Input: part model. Units: mm. Frame: model coordinates. A direction names the side the tool comes from. Give positions to 0.01 mm unless a question says otherwise; leave off trailing zeros. Write each loop counter-clockwise with the first axis right and the second up, starting at its lowest first coordinate (ties: lowest second). Pieces come first, ordered by that corner, then holes.
```python
from build123d import *

# Parameters (mm, degrees)
SALIENTE_EXTRUIR1_START      = 0.1
SALIENTE_EXTRUIR1_DEPTH      = 1.3
SALIENTE_EXTRUIR2_START      = 0.1
SALIENTE_EXTRUIR2_DEPTH      = 1.3
SALIENTE_EXTRUIR2_DEPTH_BACK = 6.6
CROQUIS2_W                   = 45.7
CROQUIS2_H                   = 27.4
CROQUIS2_R                   = 1.65
CROQUIS2_R_2                 = 1.6
SALIENTE_EXTRUIR3_DEPTH      = 5.5
REDONDEO1_R                  = 3


with BuildPart() as part:
    # Croquis1 → Saliente-Extruir1 (new body)
    with BuildSketch(Plane.XY.offset(SALIENTE_EXTRUIR1_START)):
        with BuildLine():
            Line((-105.35, -3.3), (-105.35, -9.05))
            Line((-105.35, -9.05), (-94.282475165, -9.05))
            ThreePointArc((-94.282475165, -9.05), (-93.803420224, -6.334895379), (-91.5, -7.85))
            ThreePointArc((-91.5, -7.85), (-91.634895379, -8.503420224), (-92.017524835, -9.05))
            Line((-92.017524835, -9.05), (-74.282475165, -9.05))
            ThreePointArc((-74.282475165, -9.05), (-73.803420224, -6.334895379), (-71.5, -7.85))
            ThreePointArc((-71.5, -7.85), (-71.634895379, -8.503420224), (-72.017524835, -9.05))
            Line((-72.017524835, -9.05), (-59.65, -9.05))
            Line((-59.65, -9.05), (-59.65, -3.3))
            Line((-59.65, -3.3), (-105.35, -3.3))
        make_face()
    extrude(amount=SALIENTE_EXTRUIR1_DEPTH)



with BuildPart() as body_2:
    # Croquis1<3> → Saliente-Extruir2 (new, two sides)
    with BuildSketch(Plane.XY.offset(SALIENTE_EXTRUIR2_START)) as saliente_extruir2_sk:
        with BuildLine():
            Line((-105.35, -21.65), (-105.35, -30.7))
            Line((-105.35, -30.7), (-59.65, -30.7))
            Line((-59.65, -30.7), (-59.65, -21.65))
            Line((-59.65, -21.65), (-72.017510495, -21.65))
            ThreePointArc((-72.017510495, -21.65), (-71.634891475, -22.196575296), (-71.5, -22.849986467))
            ThreePointArc((-71.5, -22.849986467), (-73.803411171, -24.365094992), (-74.282489505, -21.65))
            Line((-74.282489505, -21.65), (-92.017510495, -21.65))
            ThreePointArc((-92.017510495, -21.65), (-91.634891475, -22.196575296), (-91.5, -22.849986467))
            ThreePointArc((-91.5, -22.849986467), (-93.803411171, -24.365094992), (-94.282489505, -21.65))
            Line((-94.282489505, -21.65), (-105.35, -21.65))
        make_face()
    extrude(amount=SALIENTE_EXTRUIR2_DEPTH)
    extrude(saliente_extruir2_sk.sketch, amount=-SALIENTE_EXTRUIR2_DEPTH_BACK)


with BuildPart() as part_1:
    add(part.part)

    add(body_2.part)  # Saliente-Extruir3 merges body 2
    # Croquis2 → Saliente-Extruir3 (add)
    with BuildSketch(Plane.XY.offset(1.4)):
        with Locations((-82.5, -17)):
            Rectangle(CROQUIS2_W, CROQUIS2_H)
        with Locations(Location((-93.15, -7.85, 0), (0, 0, 226.658241773))):
            Circle(CROQUIS2_R, mode=Mode.SUBTRACT)
        with Locations(Location((-73.15, -7.85, 0), (0, 0, 226.658241773))):
            Circle(CROQUIS2_R, mode=Mode.SUBTRACT)
        with Locations(Location((-93.15, -22.849986467, 0), (0, 0, 133.342442907))):
            Circle(CROQUIS2_R, mode=Mode.SUBTRACT)
        with Locations(Location((-73.15, -22.849986467, 0), (0, 0, 133.342442907))):
            Circle(CROQUIS2_R, mode=Mode.SUBTRACT)
        with Locations((-96.65, -15.35)):
            Circle(CROQUIS2_R_2, mode=Mode.SUBTRACT)
        with Locations((-71.65, -15.35)):
            Circle(CROQUIS2_R_2, mode=Mode.SUBTRACT)
    extrude(amount=SALIENTE_EXTRUIR3_DEPTH)

    # Redondeo1
    redondeo1_edges = [part_1.edges().sort_by_distance(p)[0] for p in [
        (-59.65, -17, 6.9),
    ]]
    fillet(redondeo1_edges, radius=REDONDEO1_R)


solid = part_1.part
```
Q1. Section C-C, the plane z = 2.25. Return the cut outline in (x, y).
Q2. Access query for faces 4 (the flat face through (-66, -9.05, 1)), 5 (the flat face through (-83, -6, 0.1)), 6 (the cylindrical face through (-60.51, -16.81, 6)). Directions: +Z, -Z, +X, -X, +Y, -Y. A direction counts if a zero-diameter tool reaches every point of the face in a straight line with its end or side. Return the directions, or none.
Q3. Section B-B, the plane y = -15.35. Return the cut outline in (x, z).
Q4. Section D-D, the plane x = -64. Return the cut outline in (y, z).
Q5. Mould query, pull axis Y, two halves, no side actions, for faces 1 (the flat face through (-83, -3.3, 3)), 2 (the cylindrical face through (-70.124, -14.869, 4.111)), 3 (the flat face through (-105.35, -20, 2)). Classes: +Y half, -Y half, draft (parallel to the pull), parting line (faces both ways), or undercut.
Q6. Section A-A, the plane x = -96.65. Return the cut outline in (y, z).
Q7. Pin query (flat end, axial travel): pin 1 (4 mm diameter, centred on x = -93.15, y = -22.85, fed in from +Z); pin 2 (4.5 mm diameter, centred on x = -73.15, y = -7.85, fed in from -Z); pin 3 (4 mm diameter, centred on x = -79, y = -18, fed in from -Z); pin 4 (4 mm diameter, centred on x = -65, z = -4.5, fed in from +Y). Return the tip coordinate at first contact, or that it passes through.
Q8. Material intervals for line 1 along Y through (x, z) = (-93, 0.75); line 2 along X through (y, z) = (-14.75, 2.75); line 3 along X through (y, z) = (-22, -1.25), sorted ascending.
Solutions:
1. outline: (-105.35, -30.7) - (-59.65, -30.7) - (-59.65, -3.3) - (-105.35, -3.3) - close; hole circle Ø3.2 at (-96.65, -15.35); hole circle Ø3.3 at (-93.15, -22.85); hole circle Ø3.3 at (-93.15, -7.85); hole circle Ø3.3 at (-73.15, -22.85); hole circle Ø3.3 at (-73.15, -7.85); hole circle Ø3.2 at (-71.65, -15.35)
2. face 4: -Z, +X, -X
2. face 5: -Z, +X, -X, +Y
2. face 6: +Z, +X, +Y, -Y
3. outline: (-105.35, 1.4) - (-98.25, 1.4) - (-98.25, 6.9) - (-105.35, 6.9) - close; (-95.05, 1.4) - (-73.25, 1.4) - (-73.25, 6.9) - (-95.05, 6.9) - close; (-70.05, 1.4) - (-59.65, 1.4) - (-59.65, 3.9) arc R3 ccw to (-62.65, 6.9) - (-70.05, 6.9) - close
4. outline: (-30.7, -6.5) - (-21.65, -6.5) - (-21.65, 1.4) - (-9.05, 1.4) - (-9.05, 0.1) - (-3.3, 0.1) - (-3.3, 6.9) - (-30.7, 6.9) - close
5. face 1: +Y half
5. face 2: undercut
5. face 3: draft
6. outline: (-30.7, -6.5) - (-21.65, -6.5) - (-21.65, 1.4) - (-16.95, 1.4) - (-16.95, 6.9) - (-30.7, 6.9) - close; (-13.75, 1.4) - (-9.05, 1.4) - (-9.05, 0.1) - (-3.3, 0.1) - (-3.3, 6.9) - (-13.75, 6.9) - close
7. pin 1: stops at z = 6.9
7. pin 2: stops at z = 0.1
7. pin 3: stops at z = 1.4
7. pin 4: stops at y = -21.65
8. line 1: y = -30.7 to -24.49, -6.21 to -3.3
8. line 2: x = -105.35 to -98.13, -95.17 to -73.13, -70.17 to -59.65
8. line 3: x = -105.35 to -94.56, -91.74 to -74.56, -71.74 to -59.65
